from build123d import *

# Parameters (mm, degrees)
F1_DEPTH = 3.175
F2_DEPTH = 3.81


with BuildPart() as f1:
    # F0 (on Right) → F1 (new body)
    with BuildSketch(Plane.YZ):
        with BuildLine():
            ThreePointArc((25.4, -1.5875), (23.8125, 0), (25.4, 1.5875))
            Line((25.4, 1.5875), (-25.4, 1.5875))
            ThreePointArc((-25.4, 1.5875), (-24.277468, 1.122532), (-23.8125, 0))
            ThreePointArc((-23.8125, 0), (-24.277468, -1.122532), (-25.4, -1.5875))
            Line((-25.4, -1.5875), (25.4, -1.5875))
        make_face()
    extrude(amount=F1_DEPTH)

    # F0 (on Right) → F2 (join)
    with BuildSketch(Plane.YZ):
        with BuildLine():
            ThreePointArc((-23.8125, 0), (-24.277468, 1.122532), (-25.4, 1.5875))
            Line((-25.4, 1.5875), (-25.4, -1.5875))
            ThreePointArc((-25.4, -1.5875), (-24.277468, -1.122532), (-23.8125, 0))
        make_face()
        with BuildLine():
            Line((-25.4, -1.5875), (-25.4, 1.5875))
            ThreePointArc((-25.4, 1.5875), (-26.9875, 0), (-25.4, -1.5875))
        make_face()
        with BuildLine():
            ThreePointArc((26.9875, 0), (26.522532, 1.122532), (25.4, 1.5875))
            Line((25.4, 1.5875), (25.4, -1.5875))
            ThreePointArc((25.4, -1.5875), (26.522532, -1.122532), (26.9875, 0))
        make_face()
        with BuildLine():
            Line((25.4, -1.5875), (25.4, 1.5875))
            ThreePointArc((25.4, 1.5875), (23.8125, 0), (25.4, -1.5875))
        make_face()
    extrude(amount=F2_DEPTH)


solid = f1.part
Can you work these out from the model? Positions are in its coordinate system, mm. Round coordinates to 2 decimals unless told otherwise and drop trailing zeros. Loops run counter-clockwise (first coordinate to the right, second up) from the corner with the lowest first, then second, coordinate; pieces in that order, holes last. Notation, with made-up numbers: (-35, 52) - (-17, 52) arc R23 ccw to (-17, 82) - close; hole circle Ø1 at (57.25, 78). An arc over 180 degrees is marked (long way). Write item = value, one per line. Start each with the question number.
(1) If I drill on probe 1 along X at (y, z) = (19, -0.95) (3 decimals); probe 2 along Y at (x, z) = (2.9, -0.1); probe 3 along Y at (x, z) = (2.65, -1.3), over which ranges is the centre line in solid material (lowest first)? Write a range as [from, to].
(2) If we section it at B-B (y = -3): Please give me the cut outline in (x, z) (1 decimal).
(3) For P1, Ø1.5, axis at y = 18, z = 1, coming from the +X side (3 decimals), with a flat end and sliding along its axis, tell me the tip position at first contact or that it passes through.
(4) If we section it at A-A (z = 0.7): Please give me the cut outline in (x, y) (3 decimals).
Ans:
q1.probe_1 = [0, 3.175]
q1.probe_2 = [-26.98, 26.98]
q1.probe_3 = [-26.31, 26.31]
q2.outline = (0, -1.6) - (3.2, -1.6) - (3.2, 1.6) - (0, 1.6) - close
q3.P1 = 3.175
q4.outline = (0, -26.825) - (3.81, -26.825) - (3.81, -23.975) - (3.175, -23.975) - (3.175, 23.975) - (3.81, 23.975) - (3.81, 26.825) - (0, 26.825) - close
